For this review, take the finished solid that the model builds, in its own axes (mm). Face numbers are marked on the shaded views. Coordinates: 2 decimals unless noted, no trailing zeros.
1) Insertion check: P1, Ø3, axis at x = -65.5, y = -116.5, coming from the +Z side; P2, Ø5, axis at x = 78.5, y = -165, coming from the -Z side; P3, Ø8, axis at y = 6, z = 11, coming from the +X side. Each pin has a flat end and moves straight along its axis. Give the tip position at first contact, or say it passes through.
2) To check wall thickness, follow line 1 along Z through (x, y) = (90, -119); line 2 along X through (y, z) = (18.5, 41.5); line 3 along X through (y, z) = (-175, 50.5). State the ranges of each line that lie inside material, in increasing order.
3) Mouldability with a two-part tool opening along X and no side actions: class the marked faces 1 and 2 as pulls with the +X half, pulls with the -X half, needs draft (parallel to the pull), parting line crosses it, or undercut.
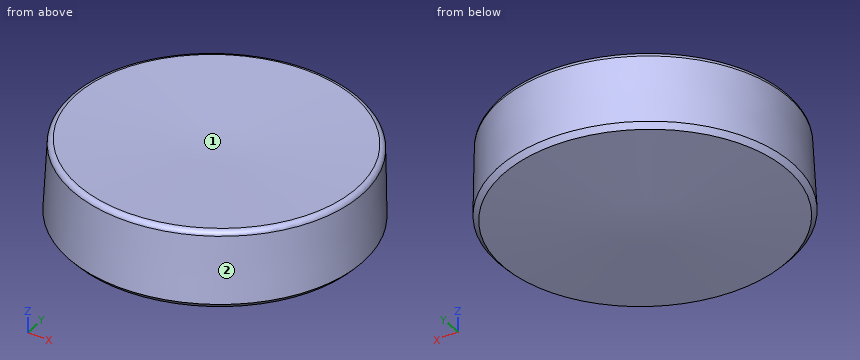
from build123d import *

# Parameters (mm, degrees)
F2_R    = 5.08
F3_SIZE = 5.08


with BuildPart() as f1:
    # F0 (on Right) → F1 (revolve)
    with BuildSketch(Plane.YZ):
        Polygon((-71.8356743455, 79.0152773261), (-74.5772719383, 0), (76.0060697794, 0), (76.0060697794, 79.0152773261), align=None)
    revolve(axis=Axis((0, -73.2064731419, 39.5076386631), (0, -0.0346761903, -0.9993986001)))

    # F2
    f2_edges = [f1.edges().sort_by_distance(p)[0] for p in [
        (0, -219.321877, 89.262288),
    ]]
    fillet(f2_edges, radius=F2_R)

    # F3
    f3_edges = [f1.edges().sort_by_distance(p)[0] for p in [
        (0, -224.798479, 10.437033),
    ]]
    chamfer(f3_edges, length=F3_SIZE)


solid = f1.part
Result:
1. P1: stops at z = 83.41
1. P2: stops at z = 7.14
1. P3: stops at x = 129.47
2. line 1: z = 5.03 to 84.18
2. line 2: x = -117.69 to 117.69
2. line 3: x = -108.57 to 108.57
3. face 1: undercut
3. face 2: parting line crosses it
